Print and shaded views of the part. All mm, measured from the part's lowest x, y and z. A direction names the side the tool comes from. Round coordinates to 2 decimals unless told otherwise and drop trailing zeros. Write each loop counter-clockwise with the first axis right and the second up, starting at its lowest first coordinate (ties: lowest second). Pieces come first, ordered by that corner, then holes. Notation, with made-up numbers: (-35.75, 72.25) - (-31.75, 72.25) arc R27 cw to (-31.75, 94.25) - close; hole circle Ø6 at (73.25, 52). An arc over 180 degrees is marked (long way). Put each result on its own line as item: value. Start each with the question number.
Item 1: 3-axis set-ups, long thin cutter, end or side, ignore diameter. For the marked faces 1 and 2: which of +Z, -Z, +X, -X, +Y, -Y reach the whole face in a straight line?
Item 2: Cut at A-A (z = 1.25). Give the cut face in (x, y) (3 decimals).
Item 3: Drill centre lines: line 1 (Z direction, x = 1.35, y = 1.55); line 2 (Z direction, x = 1.4, y = 2.15); line 3 (X direction, y = 1.2, z = 6.75). Where is each one in solid material? Low to high. Write a range as from..to.
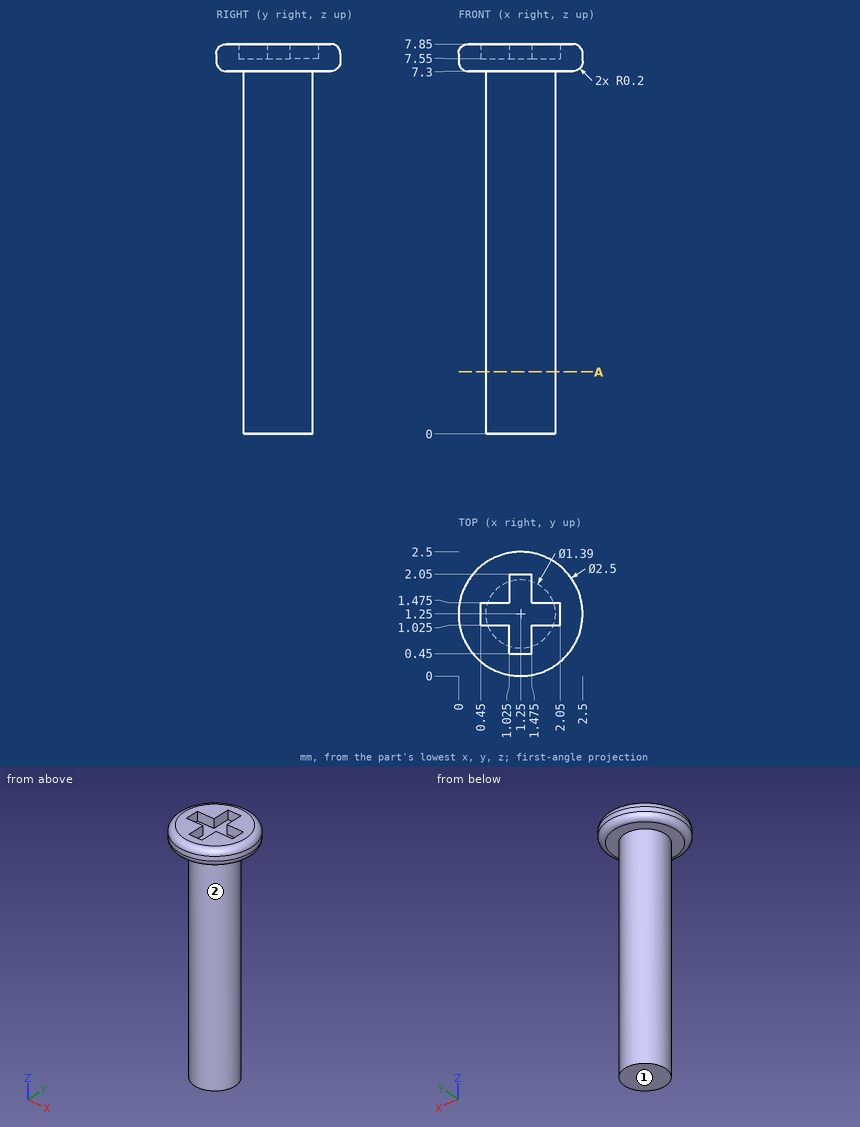
Output values:
1. face 1: -Z, +X, -X, +Y, -Y
1. face 2: -Z
2. outline: circle Ø1.39 at (1.25, 1.25)
3. line 1: 0..7.55
3. line 2: 7.3..7.85
3. line 3: 0.56..1.94
